Geometry: final body of the model. Coordinates: model frame, mm. Give positions to 0.01 mm unless a question says otherwise; leave off trailing zeros. Order: outer loops, then holes, each group sorted by start corner. A loop starts at its lowest first (then second) coordinate and runs counter-clockwise, first axis right, second up. Notation, with made-up numbers: (51, 56) -> (60, 56) arc R21 ccw to (60, 86) -> close; hole circle Ø9 at (-13, 53.5). An arc over 180 degrees is marked (long way). Write item = value, one per line.
```python
from build123d import *

# Parameters (mm, degrees)
SKETCH2_W      = 57
SKETCH2_H      = 84
SKETCH2_R      = 1.35
SKETCH2_R_2    = 0.35
SKETCH2_R_3    = 0.45
EXTRUDE1_DEPTH = 0.79375


with BuildPart() as part:
    # Sketch2 → Extrude1 (new, symmetric)
    with BuildSketch(Plane(origin=(0, 0, 0), x_dir=(1, 0, 0), z_dir=(0, 1, 0))):
        Rectangle(SKETCH2_W, SKETCH2_H)
        with Locations(Location((25.3, 38.75, 0), (0, 0, 270))):
            Circle(SKETCH2_R, mode=Mode.SUBTRACT)
        with Locations(Location((25.3, -38.75, 0), (0, 0, 270))):
            Circle(SKETCH2_R, mode=Mode.SUBTRACT)
        with Locations(Location((-25.3, -38.75, 0), (0, 0, 270))):
            Circle(SKETCH2_R, mode=Mode.SUBTRACT)
        with Locations(Location((-25.3, 38.75, 0), (0, 0, 270))):
            Circle(SKETCH2_R, mode=Mode.SUBTRACT)
        with Locations(Location((23.8, -33.07, 0), (0, 0, 270))):
            Circle(SKETCH2_R_2, mode=Mode.SUBTRACT)
        with Locations(Location((-23.8, -33.07, 0), (0, 0, 270))):
            Circle(SKETCH2_R_2, mode=Mode.SUBTRACT)
        with Locations(Location((23.8, 33.1, 0), (0, 0, 270))):
            Circle(SKETCH2_R_3, mode=Mode.SUBTRACT)
        with Locations(Location((-23.8, 33.1, 0), (0, 0, 270))):
            Circle(SKETCH2_R_3, mode=Mode.SUBTRACT)
    extrude(amount=EXTRUDE1_DEPTH, both=True)


solid = part.part
```
1) Section query B-B (x = -25.3). Output: boundary loops of the cut face in (y, z).
Check sheet entries:
outline = (-0.79, -42) -> (0.79, -42) -> (0.79, -40.1) -> (-0.79, -40.1) -> close; (-0.79, -37.4) -> (0.79, -37.4) -> (0.79, 37.4) -> (-0.79, 37.4) -> close; (-0.79, 40.1) -> (0.79, 40.1) -> (0.79, 42) -> (-0.79, 42) -> close
2) First-contact query: P1, Ø2, axis at x = 25.3, z = 38.75, coming from the +Y side. Flat tip, straight axial feed; report the tip coordinate or a pass-through.
Check sheet entries:
P1 = through
3) Section query A-A (z = 38.75). Output: boundary loops of the cut face in (x, y), plus the area to 3 significant figures.
Check sheet entries:
outline = (-28.5, -0.79) -> (-26.65, -0.79) -> (-26.65, 0.79) -> (-28.5, 0.79) -> close; (-23.95, -0.79) -> (23.95, -0.79) -> (23.95, 0.79) -> (-23.95, 0.79) -> close; (26.65, -0.79) -> (28.5, -0.79) -> (28.5, 0.79) -> (26.65, 0.79) -> close
area = 81.9 mm²
4) Line query: line 1 (Z direction, x = 23.8, y = 0.25); line 2 (X direction, y = 0.55, z = 33.07); line 3 (X direction, y = -0.6, z = 39.5). Output: solid intervals per line, ascending. Write a range as from..to.
Check sheet entries:
line_1 = -42..-33.55, -32.65..32.72, 33.42..42
line_2 = -28.5..-24.15, -23.45..23.45, 24.15..28.5
line_3 = -28.5..-26.42, -24.18..24.18, 26.42..28.5
